Here's how the part is built. I have some questions about the finished solid (model axes, mm). A direction names the side the tool comes from. Round coordinates to 2 decimals unless told otherwise and drop trailing zeros. Loops run counter-clockwise (first coordinate to the right, second up) from the corner with the lowest first, then second, coordinate; pieces in that order, holes last. Notation, with made-up numbers: M 75.5,40 L 83.5,40 A11 cw 83.5,54 Z; hole C -1,13.5 d10. An arc over 180 degrees is marked long. Use a Markdown table: item, result.
```python
from build123d import *

# Parameters (mm, degrees)
SKETCH1_R           = 4.25
SKETCH1_R_2         = 1.5
SKETCH1_W           = 40
SKETCH1_H           = 20
BOSS_EXTRUDE1_DEPTH = 6.1
SKETCH2_R           = 10.35
CUT_EXTRUDE1_DEPTH  = 2.5
SKETCH3_R           = 0.75
CUT_EXTRUDE3_DEPTH  = 3.6


with BuildPart() as part:
    # Sketch1 → Boss-Extrude1 (new body)
    with BuildSketch(Plane(origin=(0, 0, 0), x_dir=(1, 0, 0), z_dir=(0, 1, 0))):
        with BuildLine():
            Line((150, 20), (159.5, 20))
            Line((159.5, 20), (166.5, 20))
            ThreePointArc((166.5, 20), (186.5, 0), (166.5, -20))
            Line((166.5, -20), (159.5, -20))
            Line((159.5, -20), (150, -20))
            Line((150, -20), (0, -20))
            ThreePointArc((0, -20), (-20, 0), (0, 20))
            Line((0, 20), (150, 20))
        make_face()
        with Locations(Location((0, 0, 0), (0, 0, 270))):
            Circle(SKETCH1_R, mode=Mode.SUBTRACT)
        with Locations(Location((165, 4.825, 0), (0, 0, 270))):
            Circle(SKETCH1_R_2, mode=Mode.SUBTRACT)
        with Locations(Location((165, -4.825, 0), (0, 0, 270))):
            Circle(SKETCH1_R_2, mode=Mode.SUBTRACT)
        with Locations(Location((114, 4.825, 0), (0, 0, 270))):
            Circle(SKETCH1_R_2, mode=Mode.SUBTRACT)
        with Locations(Location((114, -4.825, 0), (0, 0, 270))):
            Circle(SKETCH1_R_2, mode=Mode.SUBTRACT)
        with Locations((139.5, 0)):
            Rectangle(SKETCH1_W, SKETCH1_H, mode=Mode.SUBTRACT)
    extrude(amount=BOSS_EXTRUDE1_DEPTH)

    # Sketch2 → Cut-Extrude1 (cut)
    with BuildSketch(Plane(origin=(0, 6.1, 0), x_dir=(1, 0, 0), z_dir=(0, 1, 0))):
        with Locations(Location((0, 0, 0), (0, 0, 270))):
            Circle(SKETCH2_R)
    extrude(amount=-CUT_EXTRUDE1_DEPTH, mode=Mode.SUBTRACT)

    # Sketch3 → Cut-Extrude3 (cut)
    with BuildSketch(Plane(origin=(0, 3.6, 0), x_dir=(1, 0, 0), z_dir=(0, 1, 0))):
        with Locations(Location((-7.52500865, 2.715556079, 0), (0, 0, 270))):
            Circle(SKETCH3_R)
        with Locations(Location((7.52500865, -2.715556079, 0), (0, 0, 270))):
            Circle(SKETCH3_R)
        with Locations(Location((2.715556079, 7.52500865, 0), (0, 0, 270))):
            Circle(SKETCH3_R)
        with Locations(Location((-2.715556079, -7.52500865, 0), (0, 0, 270))):
            Circle(SKETCH3_R)
    extrude(amount=-CUT_EXTRUDE3_DEPTH, mode=Mode.SUBTRACT)


solid = part.part
```
Q1. Will these pins go through, and if not, where does the flat tip stop? P1, Ø1.5, axis at x = 13.5, z = -5.5, coming from the -Y side; P2, Ø2, axis at x = -7.53, z = -2.72, coming from the +Y side.
Return value:
| item | result |
|---|---|
| P1 | stops at y = 0 |
| P2 | stops at y = 3.6 |
Q2. Imagine slicing it at A-A, the plane x = 137.5. Please give me the cut outline in (y, z).
Return value:
| item | result |
|---|---|
| outline | M 0,-20 L 6.1,-20 L 6.1,-10 L 0,-10 Z; M 0,10 L 6.1,10 L 6.1,20 L 0,20 Z |
Q3. We'd pull the mould along Z, two halves only. Please class faces 4 (the flat face through (85, 6.1, 0)), 5 (the cylindrical face through (4.214, 1.775, -0.553)), 6 (the cylindrical face through (186.495, 3.007, -0.44)), 7 (the flat face through (-4.5, 3.6, -0.1)): pulls with the +Z half, pulls with the -Z half, needs draft (parallel to the pull), parting line crosses it, or undercut.
Return value:
| item | result |
|---|---|
| face 4 | needs draft |
| face 5 | undercut |
| face 6 | parting line crosses it |
| face 7 | undercut |
Q4. For faces 1 (the cylindrical face through (-6.3, 4.87, -8.21)), 2 (the flat face through (119.5, 3, 0)), 3 (the cylindrical face through (-20, 3, 0)), which set-ups out of +Z, -Z, +X, -X, +Y, -Y let a thin tool reach every point of the face, with its end or its side?
Return value:
| item | result |
|---|---|
| face 1 | +Y |
| face 2 | +Y, -Y |
| face 3 | -X, +Y, -Y |
Q5. Imagine slicing it at B-B, the plane y = 2.25. Give the number of separate pieces and of enclosed holes in the cut face, then the cut area to 3 significant figures.
Return value:
| item | result |
|---|---|
| separate pieces | 1 |
| enclosed holes | 10 |
| area | 7,020 mm^2 |
Q6. Imagine slicing it at C-C, the plane z = -13. Please give me the cut outline in (x, y).
Return value:
| item | result |
|---|---|
| outline | M -15.2,0 L 181.7,0 L 181.7,6.1 L -15.2,6.1 Z |
Q7. I need wall thicknesses on line 1 (Z direction, x = 165, y = 4) (3 decimals); line 2 (X direction, y = 1.5, z = 0); line 3 (X direction, y = 5.1, z = 0). Which ranges of each line are inside material? Lowest first, please. Write a range as from..to.
Return value:
| item | result |
|---|---|
| line 1 | z = -20..-6.325, -3.325..3.325, 6.325..20 |
| line 2 | x = -20..-4.25, 4.25..119.5, 159.5..186.5 |
| line 3 | x = -20..-10.35, 10.35..119.5, 159.5..186.5 |
